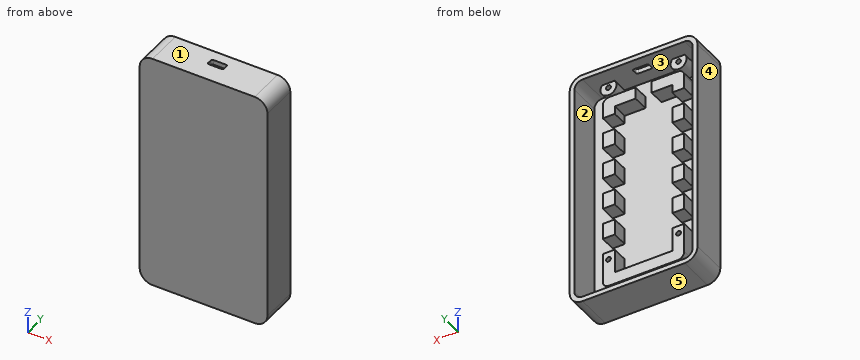
Autodesk Inventor part; units mm, degrees
ref_plane "YZ Plane" through (0, 0, 0) normal (1, 0, 0) x (0, 1, 0)
ref_plane "XZ Plane" through (0, 0, 0) normal (0, 1, 0) x (-1, 0, 0)
ref_plane "XY Plane" through (0, 0, 0) normal (0, 0, 1) x (1, 0, 0)
sketch "Sketch1" plane through (0, 0, 0) normal (0, 1, 0) x (-1, 0, 0)
  line L0 (26.7027, -40.183) -> (-37.2973, -40.183)
  line L1 (-45.2973, -32.183) -> (-45.2973, 101.817)
  line L2 (-37.2973, 109.817) -> (26.7027, 109.817)
  line L3 (34.7027, 101.817) -> (34.7027, -32.183)
  arc A0 (26.7027, -40.183) -> (34.7027, -32.183) centre (26.7027, -32.183) ccw
  arc A1 (-45.2973, -32.183) -> (-37.2973, -40.183) centre (-37.2973, -32.183) ccw
  arc A2 (-37.2973, 109.817) -> (-45.2973, 101.817) centre (-37.2973, 101.817) ccw
  arc A3 (34.7027, 101.817) -> (26.7027, 109.817) centre (26.7027, 101.817) ccw
  point P0 (0, 0)
  point P1 (-45.2973, 109.817)
  point P2 (-45.2973, -40.183)
  point P3 (34.7027, 109.817)
  dimension "d0" = 80
  dimension "d1" = 150
  dimension "d2" = 8
extrude "Extrusion1" add sketch "Sketch1" along normal blind 3
sketch "Sketch2" plane through (0, 3, 0) normal (0, 1, 0) x (1, 0, 0)
  line L0 (-26.7027, 40.183) -> (37.2973, 40.183)
  line L1 (45.2973, 32.183) -> (45.2973, -101.817)
  line L2 (37.2973, -109.817) -> (-26.7027, -109.817)
  line L3 (-34.7027, -101.817) -> (-34.7027, 32.183)
  arc A0 (-26.7027, 40.183) -> (-34.7027, 32.183) centre (-26.7027, 32.183) ccw
  arc A1 (45.2973, 32.183) -> (37.2973, 40.183) centre (37.2973, 32.183) ccw
  arc A2 (37.2973, -109.817) -> (45.2973, -101.817) centre (37.2973, -101.817) ccw
  arc A3 (-34.7027, -101.817) -> (-26.7027, -109.817) centre (-26.7027, -101.817) ccw
  line L4 (37.2973, 37.183) -> (-26.7027, 37.183)
  arc A4 (-26.7027, 37.183) -> (-31.7027, 32.183) centre (-26.7027, 32.183) ccw
  line L5 (-31.7027, 32.183) -> (-31.7027, -101.817)
  arc A5 (-31.7027, -101.817) -> (-26.7027, -106.817) centre (-26.7027, -101.817) ccw
  line L6 (-26.7027, -106.817) -> (37.2973, -106.817)
  arc A6 (37.2973, -106.817) -> (42.2973, -101.817) centre (37.2973, -101.817) ccw
  line L7 (42.2973, -101.817) -> (42.2973, 32.183)
  arc A7 (42.2973, 32.183) -> (37.2973, 37.183) centre (37.2973, 32.183) ccw
  point P0 (0, 0)
  dimension "d5" = 8
  dimension "d6" = 3
extrude "Extrusion2" add sketch "Sketch2" along normal blind 20
sketch "Sketch3" plane through (-26.7027, 0, 109.817) normal (0, 0, 1) x (1, 0, 0)
  line L0 (64, 0) -> (0, 0)
  line L1 (32, 0) -> (32, 14)
  line L2 (28, 16.25) -> (36, 16.25)
  line L3 (37, 15.25) -> (37, 12.75)
  line L4 (36, 11.75) -> (28, 11.75)
  line L5 (27, 12.75) -> (27, 15.25)
  line L6 (27, 16.25) -> (37, 11.75) construction
  line L7 (37, 16.25) -> (27, 11.75) construction
  arc A0 (28, 16.25) -> (27, 15.25) centre (28, 15.25) ccw
  arc A1 (37, 15.25) -> (36, 16.25) centre (36, 15.25) ccw
  arc A2 (36, 11.75) -> (37, 12.75) centre (36, 12.75) ccw
  arc A3 (27, 12.75) -> (28, 11.75) centre (28, 12.75) ccw
  point P0 (26.7027, 0)
  dimension "d9" = 14
  dimension "d10" = 10
  dimension "d11" = 4.5
  dimension "d14" = 1
extrude "Extrusion3" cut sketch "Sketch3" against normal blind 3
sketch "Sketch4" plane through (0, 3, 0) normal (0, 1, 0) x (1, 0, 0)
  line L0 (37.2973, 37.183) -> (-26.7027, 37.183)
  line L1 (1.2973, -106.817) -> (9.2973, -106.817)
  line L2 (-31.7027, 32.183) -> (-31.7027, -101.817)
  line L3 (-12.7027, 20.183) -> (23.2973, 20.183)
  circle A0 centre (-16.6527, 10.133) radius 1.5
  circle A1 centre (27.2473, 10.133) radius 1.5
  circle A2 centre (-16.6527, -103.767) radius 1.5
  circle A3 centre (27.2473, -103.767) radius 1.5
  line L4 (26.7973, 27.683) -> (-16.2027, 27.683)
  arc A4 (-16.2027, 27.683) -> (-20.2027, 23.683) centre (-16.2027, 23.683) ccw
  arc A5 (30.7973, 23.683) -> (26.7973, 27.683) centre (26.7973, 23.683) ccw
  arc A6 (26.7973, -97.317) -> (30.7973, -93.317) centre (26.7973, -93.317) ccw
  arc A7 (-20.2027, -93.317) -> (-16.2027, -97.317) centre (-16.2027, -93.317) ccw
  arc A8 (-12.6907, -106.817) -> (-20.6147, -106.817) centre (-16.6527, -103.767) ccw
  line L5 (-20.6147, -106.817) -> (-12.6907, -106.817)
  line L6 (-26.7027, -109.817) -> (37.2973, -109.817)
  arc A9 (31.2093, -106.817) -> (23.2853, -106.817) centre (27.2473, -103.767) ccw
  line L7 (23.2853, -106.817) -> (31.2093, -106.817)
  line L8 (-20.2027, 5.183) -> (-12.7027, 5.183)
  line L9 (23.2973, 5.183) -> (30.7973, 5.183)
  line L10 (-20.2027, -4.817) -> (-12.7027, -4.817)
  line L11 (23.2973, -4.817) -> (30.7973, -4.817)
  line L12 (-20.2027, -14.817) -> (-12.7027, -14.817)
  line L13 (23.2973, -14.817) -> (30.7973, -14.817)
  line L14 (-20.2027, -24.817) -> (-12.7027, -24.817)
  line L15 (23.2973, -24.817) -> (30.7973, -24.817)
  line L16 (-20.2027, -34.817) -> (-12.7027, -34.817)
  line L17 (23.2973, -34.817) -> (30.7973, -34.817)
  line L18 (-20.2027, -44.817) -> (-12.7027, -44.817)
  line L19 (23.2973, -44.817) -> (30.7973, -44.817)
  line L20 (-20.2027, -54.817) -> (-12.7027, -54.817)
  line L21 (23.2973, -54.817) -> (30.7973, -54.817)
  line L22 (-20.2027, -64.817) -> (-12.7027, -64.817)
  line L23 (23.2973, -64.817) -> (30.7973, -64.817)
  line L24 (-20.2027, -74.817) -> (-12.7027, -74.817)
  line L25 (23.2973, -74.817) -> (30.7973, -74.817)
  line L26 (-20.2027, -84.817) -> (-12.7027, -84.817)
  line L27 (23.2973, -84.817) -> (30.7973, -84.817)
  line L28 (-12.7027, 5.183) -> (-12.7027, 20.183)
  line L29 (-20.2027, 23.683) -> (-20.2027, 5.183)
  line L30 (23.2973, 20.183) -> (23.2973, 5.183)
  line L31 (30.7973, 5.183) -> (30.7973, 23.683)
  line L32 (-12.7027, -89.817) -> (-12.7027, -84.817)
  line L33 (-20.2027, -84.817) -> (-20.2027, -93.317)
  line L34 (23.2973, -84.817) -> (23.2973, -89.817)
  line L35 (30.7973, -93.317) -> (30.7973, -84.817)
  line L36 (-12.7027, -74.817) -> (-12.7027, -64.817)
  line L37 (-20.2027, -64.817) -> (-20.2027, -74.817)
  line L38 (23.2973, -64.817) -> (23.2973, -74.817)
  line L39 (30.7973, -74.817) -> (30.7973, -64.817)
  line L40 (30.7973, -14.817) -> (30.7973, -4.817)
  line L41 (23.2973, -4.817) -> (23.2973, -14.817)
  line L42 (-12.7027, -14.817) -> (-12.7027, -4.817)
  line L43 (-20.2027, -4.817) -> (-20.2027, -14.817)
  line L44 (-20.2027, -24.817) -> (-20.2027, -34.817)
  line L45 (-20.2027, -44.817) -> (-20.2027, -54.817)
  line L46 (-12.7027, -54.817) -> (-12.7027, -44.817)
  line L47 (-12.7027, -34.817) -> (-12.7027, -24.817)
  line L48 (23.2973, -24.817) -> (23.2973, -34.817)
  line L49 (23.2973, -44.817) -> (23.2973, -54.817)
  line L50 (30.7973, -54.817) -> (30.7973, -44.817)
  line L51 (30.7973, -34.817) -> (30.7973, -24.817)
  line L52 (0.2973, -89.817) -> (0.2973, -97.317)
  line L53 (10.2973, -89.817) -> (10.2973, -97.317)
  line L54 (23.2973, -89.817) -> (10.2973, -89.817)
  line L55 (0.2973, -89.817) -> (-12.7027, -89.817)
  line L56 (-16.2027, -97.317) -> (0.2973, -97.317)
  line L57 (10.2973, -97.317) -> (26.7973, -97.317)
  point P0 (0, 0)
  dimension "d25" = 36
  dimension "d26" = 110
  dimension "d29" = 3
  dimension "d30" = 7.5
  dimension "d31" = 4
  dimension "d32" = 3.5
  dimension "d33" = 3.5
extrude "Extrusion4" add sketch "Sketch4" along normal blind 10
properties part number "csing"
Geometry check sheet. Reference: the model listing, model coordinates, mm. Face numbers are marked on the shaded views. A direction names the side the tool comes from. Give positions to 0.01 mm unless a question says otherwise; leave off trailing zeros. Write each loop counter-clockwise with the first axis right and the second up, starting at its lowest first coordinate (ties: lowest second). Pieces come first, ordered by that corner, then holes. Notation, with made-up numbers: M 4,11 L 19,11 A23 cw 19,20 Z; hole C 51.5,-18.75 d11. An arc over 180 degrees is marked long. Answer as CSV lines item,"result". Start each with the question number.
Q1. Section check A-A, the plane z = 67. Record the cut outline in (x, y), then the cut area to 3 significant figures.
Q2. Release check for a two-part mould opening along Z. For the marked faces 3, 4 and 5 record: pulls with the +Z half, pulls with the -Z half, needs draft (parallel to the pull), parting line crosses it, or undercut.
Q3. Section check C-C, the plane x = -1.5. Record the cut outline in (y, z), then the cut area to 3 significant figures.
Q4. Material ranges on L1, parallel to X at y = 9.25, z = 66; L2, parallel to Z at x = 0, y = 3.5; L3, parallel to Z at x = 6.5, y = 5, recorded low to high.
Q5. Section check D-D, the plane y = 10.25. Give the number of separate pieces and of enclosed holes in the cut face, then the cut area to 3 significant figures.
Q6. Go/stop test with flat-tipped pins: pin 1 (2 mm diameter, centred on x = -15, z = 49.5, fed in from +Y); pin 2 (5 mm diameter, centred on x = -1, z = 9, fed in from +Y). Record where each tip stops, or that it passes through.
Q7. Tool access check on the marked faces 1 and 2. Record the directions out of +Z, -Z, +X, -X, +Y, -Y that give a thin tool (end or side, any length) a straight path to the whole face; none if there is none.
Q8. Section check B-B, the plane y = 18.5. Record the cut outline in (x, z), then the cut area to 3 significant figures.
Geometry says:
1,outline,"M -34.7,0 L 45.3,0 L 45.3,23 L 42.3,23 L 42.3,3 L 30.8,3 L 30.8,13 L 23.3,13 L 23.3,3 L -12.7,3 L -12.7,13 L -20.2,13 L -20.2,3 L -31.7,3 L -31.7,23 L -34.7,23 Z"
1,area,"510 mm^2"
2,face 3,"undercut"
2,face 4,"needs draft"
2,face 5,"pulls with the -Z half"
3,outline,"M 0,-40.18 L 23,-40.18 L 23,-37.18 L 3,-37.18 L 3,-27.68 L 13,-27.68 L 13,-20.18 L 3,-20.18 L 3,89.82 L 13,89.82 L 13,97.32 L 3,97.32 L 3,106.82 L 23,106.82 L 23,109.82 L 0,109.82 Z"
3,area,"720 mm^2"
4,L1,"-34.7 to -31.7, -20.2 to -12.7, 23.3 to 30.8, 42.3 to 45.3"
4,L2,"-40.18 to -37.18, -27.68 to -20.18, 89.82 to 97.32, 106.82 to 109.82"
4,L3,"-40.18 to -37.18, -27.68 to -20.18, 106.82 to 109.82"
5,separate pieces,"12"
5,enclosed holes,"5"
5,area,"2,990 mm^2"
6,pin 1,"y = 13"
6,pin 2,"y = 3"
7,face 1,"+Z, +X, -X, +Y, -Y"
7,face 2,"+Y"
8,outline,"M -34.7,-32.18 A8 ccw -26.7,-40.18 L 37.3,-40.18 A8 ccw 45.3,-32.18 L 45.3,101.82 A8 ccw 37.3,109.82 L -26.7,109.82 A8 ccw -34.7,101.82 Z; hole M -31.7,-32.18 A5 ccw -26.7,-37.18 L 37.3,-37.18 A5 ccw 42.3,-32.18 L 42.3,101.82 A5 ccw 37.3,106.82 L -26.7,106.82 A5 ccw -31.7,101.82 Z"
8,area,"1,310 mm^2"
